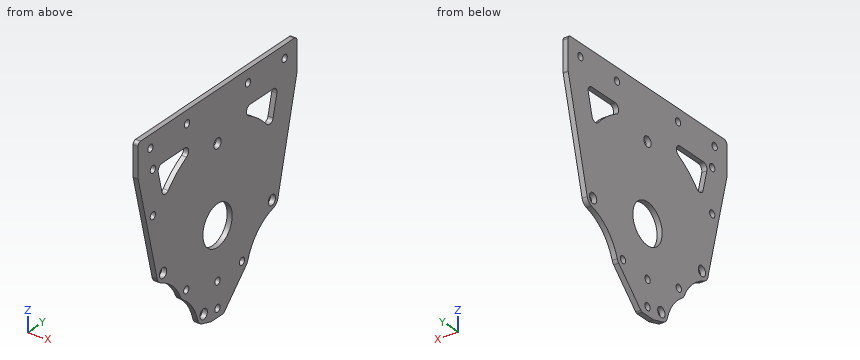
```python
from build123d import *

# Parameters (mm, degrees)
SKETCH_1_R          = 2.15
SKETCH_1_R_2        = 12
SKETCH_1_R_3        = 3
EXTRUDE_1_DEPTH     = 3
CUT_EXTRUDE_1_DEPTH = 3
FILLET_1_R          = 2
FILLET_2_R          = 2
FILLET_3_R          = 3


with BuildPart() as part:
    # ｽｹｯﾁ1 → ﾎﾞｽ - 押し出し1 (new body)
    with BuildSketch(Plane(origin=(0, 0, 0), x_dir=(0, 0, -1), z_dir=(1, 0, 0))):
        with BuildLine():
            Line((0, 0), (20, 0))
            Line((20, 0), (81.721631315, 15.55153458))
            ThreePointArc((81.721631315, 15.55153458), (83.805915962, 16.648877548), (85.156498305, 18.57873024))
            ThreePointArc((85.156498305, 18.57873024), (91.240951268, 28.202978223), (100.473591964, 34.86669062))
            ThreePointArc((100.473591964, 34.86669062), (101.625387424, 35.607613327), (102.53294649, 36.633252532))
            ThreePointArc((102.53294649, 36.633252532), (109.848876527, 44.266796828), (119.358709974, 48.888149295))
            ThreePointArc((119.358709974, 48.888149295), (121.530071674, 50.159012288), (122.807632728, 52.326439826))
            Line((122.807632728, 52.326439826), (125, 60))
            Line((125, 60), (125, 70))
            Line((125, 70), (106.736076333, 88.580227744))
            ThreePointArc((106.736076333, 88.580227744), (105.828986144, 89.309735766), (104.777796911, 89.809731531))
            ThreePointArc((104.777796911, 89.809731531), (92.392887273, 97.853140314), (85.346092725, 110.831009869))
            ThreePointArc((85.346092725, 110.831009869), (84.032111964, 113.138952539), (81.721631315, 114.44846542))
            Line((81.721631315, 114.44846542), (20, 130))
            Line((20, 130), (0, 130))
            Line((0, 130), (0, 0))
        make_face()
        with Locations((7.5, 120)):
            Circle(SKETCH_1_R, mode=Mode.SUBTRACT)
        with Locations((7.5, 90)):
            Circle(SKETCH_1_R, mode=Mode.SUBTRACT)
        with Locations(Location((7.5, 40, 0), (0, 0, 180))):
            Circle(SKETCH_1_R, mode=Mode.SUBTRACT)
        with Locations(Location((7.5, 10, 0), (0, 0, 180))):
            Circle(SKETCH_1_R, mode=Mode.SUBTRACT)
        with Locations((74.5, 65)):
            Circle(SKETCH_1_R_2, mode=Mode.SUBTRACT)
        with Locations((29.5, 65)):
            Circle(SKETCH_1_R_3, mode=Mode.SUBTRACT)
        with Locations((80.5, 20.4)):
            Circle(SKETCH_1_R_3, mode=Mode.SUBTRACT)
        with Locations((118, 53.7)):
            Circle(SKETCH_1_R_3, mode=Mode.SUBTRACT)
        with Locations((80.5, 109.6)):
            Circle(SKETCH_1_R_3, mode=Mode.SUBTRACT)
        with Locations((103.17032155, 85.075175272)):
            Circle(SKETCH_1_R, mode=Mode.SUBTRACT)
        with Locations((98.369942602, 39.402620443)):
            Circle(SKETCH_1_R, mode=Mode.SUBTRACT)
        with Locations((105, 65)):
            Circle(SKETCH_1_R, mode=Mode.SUBTRACT)
        with Locations((120, 65)):
            Circle(SKETCH_1_R, mode=Mode.SUBTRACT)
        with Locations((20, 12)):
            Circle(SKETCH_1_R, mode=Mode.SUBTRACT)
        with Locations((45.4, 12)):
            Circle(SKETCH_1_R, mode=Mode.SUBTRACT)
    extrude(amount=EXTRUDE_1_DEPTH)

    # ｽｹｯﾁ2 → ｶｯﾄ - 押し出し1 (cut)
    with BuildSketch(Plane(origin=(3, 0, 0), x_dir=(0, 0, -1), z_dir=(1, 0, 0))):
        with BuildLine():
            Line((20, 114.531188015), (20, 72.399324293))
            ThreePointArc((20, 72.399324293), (27.112840869, 92.918759813), (41.614001532, 109.085270837))
            Line((41.614001532, 109.085270837), (20, 114.531188015))
        make_face()
        with BuildLine():
            Line((20, 15.468811985), (41.614001532, 20.914729163))
            ThreePointArc((41.614001532, 20.914729163), (27.112840869, 37.081240187), (20, 57.600675707))
            Line((20, 57.600675707), (20, 15.468811985))
        make_face()
    extrude(amount=-CUT_EXTRUDE_1_DEPTH, mode=Mode.SUBTRACT)

    # ﾌｨﾚｯﾄ1
    fillet_1_edges = [part.edges().sort_by_distance(p)[0] for p in [
        (1.5, 130, 0),
        (1.5, 130, -20),
        (1.5, 0, -20),
        (1.5, 0, 0),
    ]]
    fillet(fillet_1_edges, radius=FILLET_1_R)

    # ﾌｨﾚｯﾄ2
    fillet_2_edges = [part.edges().sort_by_distance(p)[0] for p in [
        (1.5, 70, -125),
        (1.5, 60, -125),
    ]]
    fillet(fillet_2_edges, radius=FILLET_2_R)

    # ﾌｨﾚｯﾄ3
    fillet_3_edges = [part.edges().sort_by_distance(p)[0] for p in [
        (1.5, 114.531188015, -20),
        (1.5, 109.085270837, -41.614001532),
        (1.5, 72.399324293, -20),
        (1.5, 15.468811985, -20),
        (1.5, 57.600675707, -20),
        (1.5, 20.914729163, -41.614001532),
    ]]
    fillet(fillet_3_edges, radius=FILLET_3_R)


solid = part.part
```
Could you check a few things on this model? Use its own coordinates, in mm. Round coordinates to 2 decimals unless told otherwise and drop trailing zeros. Write each loop counter-clockwise with the first axis right and the second up, starting at its lowest first coordinate (ties: lowest second). Pieces come first, ordered by that corner, then holes. Notation, with made-up numbers: M 30.25,77.25 L 42.25,77.25 A30 ccw 42.25,105.25 Z; hole C 25,44 d5. An arc over 180 degrees is marked long. Answer in a Markdown table with one row per item. Add a question column.
Q1. Imagine slicing it at B-B (y = 120). Please give me the cut outline in (x, z), then the cut area to 3 significant figures.
Q2. Imagine slicing it at D-D (z = -30.5). Please give me the cut outline in (x, y), then the cut area to 3 significant figures.
Q3. Imagine slicing it at A-A (z = -7.5). Please give me the cut outline in (x, y), then the cut area to 3 significant figures.
Q4. If I drill on line 1 (Y direction, x = 0.6, z = -36.5); line 2 (Y direction, x = 1.1, z = -29.5); line 3 (Z direction, x = 1.2, y = 40), over which ranges is the centre line in solid material (lowest first)? Write a range as from..to.
Q5. Imagine slicing it at C-C (z = -71.5). Please give me the cut outline in (x, y).
Q6. Will these pins go through, and if not, where does the flat tip stop? pin 1 Ø5.5 at (y, z) = (10, -7.5) entering from -X; pin 2 Ø14.5 at (y, z) = (65, -74.5) entering from -X.
Values:
| question | item | result |
|---|---|---|
| 1 | outline | M 0,-59.69 L 3,-59.69 L 3,-9.65 L 0,-9.65 Z; M 0,-5.35 L 3,-5.35 L 3,0 L 0,0 Z |
| 1 | area | 166 mm^2 |
| 2 | outline | M 0,2.65 L 3,2.65 L 3,18.11 L 0,18.11 Z; M 0,32 L 3,32 L 3,62.17 L 0,62.17 Z; M 0,67.83 L 3,67.83 L 3,98 L 0,98 Z; M 0,111.89 L 3,111.89 L 3,127.35 L 0,127.35 Z |
| 2 | area | 274 mm^2 |
| 3 | outline | M 0,0 L 3,0 L 3,7.85 L 0,7.85 Z; M 0,12.15 L 3,12.15 L 3,37.85 L 0,37.85 Z; M 0,42.15 L 3,42.15 L 3,87.85 L 0,87.85 Z; M 0,92.15 L 3,92.15 L 3,117.85 L 0,117.85 Z; M 0,122.15 L 3,122.15 L 3,130 L 0,130 Z |
| 3 | area | 338 mm^2 |
| 4 | line 1 | 4.16..19.7, 25.24..104.76, 110.3..125.84 |
| 4 | line 2 | 2.39..17.86, 33.38..62, 68..96.62, 112.14..127.61 |
| 4 | line 3 | -105.14..-100.44, -96.3..-25.49, -20.51..-9.65, -5.35..0 |
| 5 | outline | M 0,12.98 L 3,12.98 L 3,53.38 L 0,53.38 Z; M 0,76.62 L 3,76.62 L 3,117.02 L 0,117.02 Z |
| 6 | pin 1 | x = 0 |
| 6 | pin 2 | through |
